Work out the finished part from the listing and answer in its coordinate system (mm). A direction names the side the tool comes from. Coordinates: 2 decimals unless noted, no trailing zeros. Loops run counter-clockwise (first coordinate to the right, second up) from the corner with the lowest first, then second, coordinate; pieces in that order, holes last. Notation, with made-up numbers: (23.5, -4.5) -> (76.5, -4.5) arc R21 ccw to (76.5, 13.5) -> close; hole circle Ø5 at (43, 73). An arc over 180 degrees is marked (long way). Answer as CSV lines item,"result".
```python
from build123d import *

# Parameters (mm, degrees)
SK_DISC_R          = 52
EXT_DISC_DEPTH     = 12
SK_C16_R           = 8
CUT_C16_DEPTH      = 12
CHAMFER_C1_SIZE    = 1
SK_BOLT88_R        = 2.75
CUT_BOLT88_DEPTH   = 12
SK_GROOVE70_R      = 36.9
SK_GROOVE70_R_2    = 33.1
CUT_GROOVE70_DEPTH = 2.4


with BuildPart() as part:
    # Sk_disc → Ext_disc (new body)
    with BuildSketch(Plane.XY):
        Circle(SK_DISC_R)
    extrude(amount=EXT_DISC_DEPTH)

    # Sk_c16 → Cut_c16 (cut)
    with BuildSketch(Plane.XY):
        Circle(SK_C16_R)
    extrude(amount=CUT_C16_DEPTH, mode=Mode.SUBTRACT)

    # Chamfer_C1
    chamfer_c1_edges = [part.edges().sort_by_distance(p)[0] for p in [
        (-52, 0, 0),
        (-52, 0, 12),
        (-8, 0, 0),
        (-8, 0, 12),
    ]]
    chamfer(chamfer_c1_edges, length=CHAMFER_C1_SIZE)

    # Sk_bolt88 → Cut_bolt88 (cut)
    with BuildSketch(Plane.XY):
        with Locations((44, 0)):
            Circle(SK_BOLT88_R)
        with Locations((22, 38.1051)):
            Circle(SK_BOLT88_R)
        with Locations((-22, 38.1051)):
            Circle(SK_BOLT88_R)
        with Locations((-44, 0)):
            Circle(SK_BOLT88_R)
        with Locations((-22, -38.1051)):
            Circle(SK_BOLT88_R)
        with Locations((22, -38.1051)):
            Circle(SK_BOLT88_R)
    extrude(amount=CUT_BOLT88_DEPTH, mode=Mode.SUBTRACT)

    # Sk_seat → Cut_seatR40 (revolve, cut)
    with BuildSketch(Plane(origin=(0, 0, 0), x_dir=(1, 0, 0), z_dir=(0, 1, 0)), mode=Mode.PRIVATE) as cut_seatr40_sk:
        with BuildLine():
            Line((10, -4.0888), (10, 0))
            Line((10, 0), (20, 0))
            ThreePointArc((20, 0), (15.138690108, -2.383595138), (10, -4.0888))
        make_face()
    revolve(cut_seatr40_sk.sketch.rotate(Axis((0, 0, 0), (0, 0, 1)), 180), axis=Axis((0, 0, 0), (0, 0, 1)), mode=Mode.SUBTRACT)

    # Sk_groove70 → Cut_groove70 (cut)
    with BuildSketch(Plane.XY):
        Circle(SK_GROOVE70_R)
        Circle(SK_GROOVE70_R_2, mode=Mode.SUBTRACT)
    extrude(amount=CUT_GROOVE70_DEPTH, mode=Mode.SUBTRACT)


solid = part.part
```
(1) For a pull along Y with two mould halves and no side action, classify faces 3 (the face through (11, 1, 12)), 4 (the face through (-41.265, -31.641, 5.93)), 5 (the face through (-24.18, 36.43, 5.92)) as pulls with the +Y half, pulls with the -Y half, needs draft (parallel to the pull), parting line crosses it, or undercut.
Computed values:
face 3,"needs draft"
face 4,"parting line crosses it"
face 5,"undercut"
(2) Consider line 1 along X through (y, z) = (-21, 0.5); line 2 along Z through (x, y) = (35, -5); line 3 along X through (y, z) = (23.5, 2). Determine where each line is inside the solid, lowest interval first.
Computed values:
line 1,"-47.02 to -30.34, -25.59 to 25.59, 30.34 to 47.02"
line 2,"2.4 to 12"
line 3,"-46.39 to -28.45, -23.31 to 23.31, 28.45 to 46.39"
(3) Flat-ended cylindrical pins translate along their axes: pin 1 Ø6 at (y, z) = (30.5, 8) entering from -X; pin 2 Ø2 at (x, z) = (-27.5, 7) entering from -Y; pin 3 Ø2 at (y, z) = (-22.5, 6.5) entering from -X. Find the tip coordinate at first contact, or state that the pin passes through.
Computed values:
pin 1,"x = -44.13"
pin 2,"y = -44.74"
pin 3,"x = -47.35"
(4) A cutting plane is placed at B-B, the plane y = 0. Count the separate pieces of the cut face and the enclosed holes in it, and give its area (3 significant figures).
Computed values:
separate pieces,"4"
enclosed holes,"0"
area,"856 mm2"
(5) A cutting plane is placed at A-A, the plane z = 6.75. Write down the section's boundary in (x, y), and give its area (3 significant figures).
Computed values:
outline,"circle Ø104 at (0, 0); hole circle Ø5.5 at (-44, 0); hole circle Ø5.5 at (-22, -38.11); hole circle Ø5.5 at (-22, 38.11); hole circle Ø16 at (0, 0); hole circle Ø5.5 at (22, -38.11); hole circle Ø5.5 at (22, 38.11); hole circle Ø5.5 at (44, 0)"
area,"8,150 mm2"
(6) Which of the six approach directions +Z, -Z, +X, -X, +Y, -Y give full straight-line access (tool end or side, diameter ignored) to faces 1 (the face through (-7.18, -32.31, 1.18)), 2 (the face through (19.82, 36.43, 5.92))?
Computed values:
face 1,"-Z"
face 2,"+Z, -Z"
